Autodesk Inventor part; units mm, degrees
ref_plane "YZ Plane" through (0, 0, 0) normal (1, 0, 0) x (0, 1, 0)
ref_plane "XZ Plane" through (0, 0, 0) normal (0, 1, 0) x (-1, 0, 0)
ref_plane "XY Plane" through (0, 0, 0) normal (0, 0, 1) x (1, 0, 0)
sketch "Sketch1" plane through (0, 0, 0) normal (0, 0, 1) x (1, 0, 0)
  line L0 (-141.4214, 0) -> (-17.9605, 123.4608)
  line L1 (17.9605, 123.4608) -> (141.4214, 0)
  line L2 (141.4214, 0) -> (0, -141.4214)
  line L3 (0, -141.4214) -> (-141.4214, 0)
  line L4 (-141.4214, 0) -> (141.4214, 0) construction
  line L5 (0, 141.4214) -> (0, -141.4214) construction
  line L6 (17.9605, 123.4608) -> (-17.9605, 123.4608)
  line L7 (-18.0434, 123.6608) -> (18.0434, 123.6608)
  line L8 (18.0434, 123.6608) -> (141.7042, 0)
  line L9 (141.7042, 0) -> (0, -141.7042)
  line L10 (0, -141.7042) -> (-141.7042, 0)
  line L11 (-141.7042, 0) -> (-18.0434, 123.6608)
  point P0 (0, 0)
  dimension "d0" = 200
  dimension "d1" = 200
  dimension "d7" = 25.4
  dimension "d8" = 25.4
  dimension "d9" = 0.2
extrude "Extrusion1" add sketch "Sketch1" along normal mid plane 10
sketch "Sketch4" plane through (-18.0434, 123.6608, 5) normal (0, 1, 0) x (1, 0, 0)
  line L0 (16.0434, 0) -> (20.0434, 0)
  line L1 (20.0434, 0) -> (20.0434, 2)
  line L2 (20.0434, 2) -> (16.0434, 2)
  line L3 (16.0434, 2) -> (16.0434, 0)
  line L4 (36.0867, 0) -> (0, 0)
  point P0 (18.0434, 5)
  point P1 (18.0434, 0)
  dimension "d16" = 4
  dimension "d17" = 2
extrude "Extrusion3" cut sketch "Sketch4" against normal up to surface (0.2 mm away)
sketch "Sketch2" plane through (0, 0, 5) normal (0, 0, 1) x (1, 0, 0)
  line L0 (141.7042, 0) -> (0, -141.7042)
  line L1 (18.0434, 123.6608) -> (141.7042, 0)
  line L2 (-18.0434, 123.6608) -> (18.0434, 123.6608)
  line L3 (-141.7042, 0) -> (-18.0434, 123.6608)
  line L4 (0, -141.7042) -> (-141.7042, 0)
extrude "Extrusion2" add sketch "Sketch2" along normal blind 0.2
mirror "Mirror1" about plane through (0, 0, 0) normal (0, 0, 1) of "Extrusion2"
equation "\"d0\" = ScintillatorWidth"
equation "\"d1\" = ScintillatorHeight"
equation "\"d7\" = cornerChamfer"
equation "\"d8\" = d7"
equation "\"d9\" = silveringThickness"
equation "\"d3\" = ScintillatorThickness"
equation "\"d5\" = silveringThickness"
equation "\"ScintillatorThickness\" = 10"
equation "\"OpticalFiberClearence\" = 0.15"
equation "\"ScintillatorEdgeClearence\" = 3"
equation "\"ScintillatorWidth\" = 200"
equation "\"ScintillatorHeight\" = 200"
equation "\"ShallowTrackDepth\" = 1.3"
equation "\"DeepTrackDepth\" = 5.571"
equation "\"FiberEdgeOffsett\" = 5"
equation "\"LoopLargeTrackRatio\" = 1.5"
equation "\"FiberSensorClerence\" = 0.5"
equation "\"MountingScrewOffsett\" = 9"
equation "\"FoilThickness\" = 0.2"
equation "\"silveringThickness\" = 0.2"
equation "\"mppcMountDepth\" = 6.35"
equation "\"opticalFiberClearence\" = 0.071"
equation "\"scintillatorEdgeClearence\" = 3"
equation "\"fiberEdgeOffsett\" = 5"
equation "\"shallowTrackDepth\" = 1.142"
equation "\"deepTrackDepth\" = 5.571"
equation "\"opticalFiberDiameter\" = 1"
equation "\"mountingSpacing\" = 18"
equation "\"cornerChamfer\" = 25.4"
equation "\"SmallTrackDiameter\" = 175"
properties part number "silvering" material "Silver"
Geometry: final body of the model. Coordinates: model frame, mm. A direction names the side the tool comes from. Give positions to 0.01 mm unless a question says otherwise; leave off trailing zeros. Write each loop counter-clockwise with the first axis right and the second up, starting at its lowest first coordinate (ties: lowest second). Pieces come first, ordered by that corner, then holes. Notation, with made-up numbers: (65.5, 23) -> (99.5, 23) arc R13 cw to (99.5, 39) -> close; hole circle Ø3 at (-11, 67). An arc over 180 degrees is marked (long way). Answer in a Markdown table with one row per item.
(1) Set-up query: faces 4 (the flat face through (-80.555, 60.866, -0.07)), 5 (the flat face through (80.739, 60.965, 0.073)). Return all of +Z, -Z, +X, -X, +Y, -Y with unobstructed straight access to the full face (end or side cutting, diameter ignored); none if empty.
Answers below:
| item | result |
|---|---|
| face 4 | none |
| face 5 | +Z, -Z, +X, +Y |
(2) Draft query along X for faces 1 (the flat face through (78.83, 62.59, -0.07)), 2 (the flat face through (2, -7, -5.2)), 3 (the flat face through (69.86, -71.844, 0.073)). Return one class per face: +X half, -X half, draft (parallel to the pull), parting line (faces both ways), or undercut.
Answers below:
| item | result |
|---|---|
| face 1 | undercut |
| face 2 | draft |
| face 3 | +X half |
(3) Section query B-B on y = -51. Return loops of the section in (x, z).
Answers below:
| item | result |
|---|---|
| outline | (-90.7, -5.2) -> (90.7, -5.2) -> (90.7, 5.2) -> (-90.7, 5.2) -> close; hole (-90.42, -5) -> (90.42, -5) -> (90.42, 5) -> (-90.42, 5) -> close |
(4) Section query C-C on x = -93. Return loops of the section in (y, z).
Answers below:
| item | result |
|---|---|
| outline | (-48.7, -5.2) -> (48.7, -5.2) -> (48.7, 5.2) -> (-48.7, 5.2) -> close; hole (-48.42, -5) -> (48.42, -5) -> (48.42, 5) -> (-48.42, 5) -> close |
(5) Pin query (flat end, axial travel): pin 1 (1 mm diameter, centred on x = -94.5, z = 1.5, fed in from +Y); pin 2 (6 mm diameter, centred on y = 90, z = 3, fed in from -X); pin 3 (4 mm diameter, centred on y = 11, z = 4, fed in from +X). Return the tip coordinate at first contact, or that it passes through.
Answers below:
| item | result |
|---|---|
| pin 1 | y = 47.7 |
| pin 2 | x = -54.7 |
| pin 3 | x = 132.7 |
(6) Section query A-A on z = -2.25. Return loops of the section in (x, y), then the cut area to 3 significant figures.
Answers below:
| item | result |
|---|---|
| outline | (-141.7, 0) -> (0, -141.7) -> (141.7, 0) -> (18.04, 123.66) -> (-18.04, 123.66) -> close; hole (-141.42, 0) -> (0, -141.42) -> (141.42, 0) -> (17.96, 123.46) -> (-17.96, 123.46) -> close |
| area | 157 mm^2 |
(7) Ray query, line 1 along Z through (x, y) = (-6.5, 108); line 2 along X through (y, z) = (-105, 1); line 3 along Y through (x, z) = (-128.5, 4). Return the intervals inside material, ascending. Write a range as [from, to].
Answers below:
| item | result |
|---|---|
| line 1 | [-5.2, -5], [5, 5.2] |
| line 2 | [-36.7, -36.42], [36.42, 36.7] |
| line 3 | [-13.2, -12.92], [12.92, 13.2] |
